For this review, take the finished solid that the model builds, in its own axes (mm). Coordinates: 2 decimals unless noted, no trailing zeros. Loops run counter-clockwise (first coordinate to the right, second up) from the corner with the lowest first, then second, coordinate; pieces in that order, holes last. Notation, with made-up numbers: (82, 87.5) -> (131, 87.5) arc R13 cw to (131, 105.5) -> close; hole circle Ø9 at (28, -19). An arc over 180 degrees is marked (long way). One line per item, written item: value.
from build123d import *

# Parameters (mm, degrees)
SKETCH1_R           = 14
BOSS_EXTRUDE1_DEPTH = 10
SKETCH2_R           = 1.5
SKETCH2_R_2         = 6
CUT_EXTRUDE1_DEPTH  = 11


with BuildPart() as part:
    # Sketch1 → Boss-Extrude1 (new body)
    with BuildSketch(Plane(origin=(0, 0, 0), x_dir=(1, 0, 0), z_dir=(0, 1, 0))):
        Circle(SKETCH1_R)
    extrude(amount=BOSS_EXTRUDE1_DEPTH)

    # Sketch2 → Cut-Extrude1 (cut, through all)
    with BuildSketch(Plane(origin=(0, 10, 0), x_dir=(1, 0, 0), z_dir=(0, 1, 0))):
        with Locations((0, 10.5)):
            Circle(SKETCH2_R)
        Circle(SKETCH2_R_2)
        with Locations((9.09326674, 5.25)):
            Circle(SKETCH2_R)
        with Locations((9.09326674, -5.25)):
            Circle(SKETCH2_R)
        with Locations((0, -10.5)):
            Circle(SKETCH2_R)
        with Locations((-9.09326674, -5.25)):
            Circle(SKETCH2_R)
        with Locations((-9.09326674, 5.25)):
            Circle(SKETCH2_R)
    extrude(amount=-CUT_EXTRUDE1_DEPTH, mode=Mode.SUBTRACT)


solid = part.part
1. Take a section at D-D, the plane x = 8. Give the boundary of the cut face in (y, z).
Return value:
outline: (0, -11.49) -> (10, -11.49) -> (10, -6.28) -> (0, -6.28) -> close; (0, -4.22) -> (10, -4.22) -> (10, 4.22) -> (0, 4.22) -> close; (0, 6.28) -> (10, 6.28) -> (10, 11.49) -> (0, 11.49) -> close
2. Insertion check: pin 1 Ø1 at (x, y) = (-5, 1) entering from -Z; pin 2 Ø4 at (x, y) = (-4.5, 8.5) entering from +Z (3 decimals); pin 3 Ø1 at (y, z) = (2.5, 2) entering from +X. Each pin has a flat end and moves straight along its axis. Give the tip position at first contact, or say it passes through.
Return value:
pin 1: stops at z = -13.26
pin 2: stops at z = 13.775
pin 3: stops at x = 13.92
3. Take a section at C-C, the plane y = 1.75. Give the boundary of the cut face in (x, z), and give its area (3 significant figures).
Return value:
outline: circle Ø28 at (0, 0); hole circle Ø3 at (-9.09, -5.25); hole circle Ø3 at (-9.09, 5.25); hole circle Ø12 at (0, 0); hole circle Ø3 at (0, -10.5); hole circle Ø3 at (0, 10.5); hole circle Ø3 at (9.09, -5.25); hole circle Ø3 at (9.09, 5.25)
area: 460 mm2
4. The part is to be moulded in two halves that separate along X. For faces 1 (the flat face through (6, 10, 3)), 2 (the cylindrical face through (0, 5, -9)), 3 (the cylindrical face through (12.932, 4.93, 5.362)), say which applies: pulls with the +X half, pulls with the -X half, needs draft (parallel to the pull), parting line crosses it, or undercut.
Return value:
face 1: needs draft
face 2: undercut
face 3: parting line crosses it
5. To check wall thickness, follow probe 1 along Z at (x, y) = (0, 3); probe 2 along X at (y, z) = (3.25, 0); probe 3 along X at (y, z) = (3.25, 5.25). State the ranges of each line that lie inside material, in increasing order. Write a range as from..to.
Return value:
probe 1: z = -14..-12, -9..-6, 6..9, 12..14
probe 2: x = -14..-6, 6..14
probe 3: x = -12.98..-10.59, -7.59..-2.9, 2.9..7.59, 10.59..12.98
6. Take a section at B-B, the plane x = 0. Give the boundary of the cut face in (y, z).
Return value:
outline: (0, -14) -> (10, -14) -> (10, -12) -> (0, -12) -> close; (0, -9) -> (10, -9) -> (10, -6) -> (0, -6) -> close; (0, 6) -> (10, 6) -> (10, 9) -> (0, 9) -> close; (0, 12) -> (10, 12) -> (10, 14) -> (0, 14) -> close
7. Take a section at A-A, the plane z = 0. Give the boundary of the cut face in (x, y).
Return value:
outline: (-14, 0) -> (-6, 0) -> (-6, 10) -> (-14, 10) -> close; (6, 0) -> (14, 0) -> (14, 10) -> (6, 10) -> close
